Design review of the part built by this model. Coordinates are the model's own, in mm. A direction names the side the tool comes from. Round coordinates to 2 decimals unless told otherwise and drop trailing zeros. Order: outer loops, then holes, each group sorted by start corner. A loop starts at its lowest first (then second) coordinate and runs counter-clockwise, first axis right, second up. Notation, with made-up numbers: M 6,-20 L 41,-20 A29 ccw 41,12 Z; hole C -1.75,80 d5. An arc over 180 degrees is marked long. Write item = value, one per line. Start each with the question number.
```python
from build123d import *

# Parameters (mm, degrees)
F0_R     = 1.5875
F0_R_2   = 3.175
F1_DEPTH = 3.048


with BuildPart() as f1:
    # F0 (on Front) → F1 (new body)
    with BuildSketch(Plane.XZ):
        with BuildLine():
            ThreePointArc((45.0512324214, 0), (42.8445348199, 5.4919768863), (37.4514062495, 7.9303141575))
            ThreePointArc((37.4514062495, 7.9303141575), (29.1762324214, 0), (37.4514062495, -7.9303141575))
            ThreePointArc((37.4514062495, -7.9303141575), (42.8445348199, -5.4919768863), (45.0512324214, 0))
        make_face()
        with BuildLine():
            ThreePointArc((9.4553399063, 115.449857494), (9.507569027, 114.875982809), (9.525, 114.3))
            ThreePointArc((9.525, 114.3), (0.0975597085, 104.7754996402), (-9.5230014915, 114.1048908181))
            Line((-9.5230014915, 114.1048908181), (-15.7463614541, 65.5168604207))
            ThreePointArc((-15.7463614541, 65.5168604207), (0.016359288, 79.3749915708), (15.7504847833, 65.484402704))
            Line((15.7504847833, 65.484402704), (9.4553399063, 115.449857494))
        make_face()
        with Locations((-6.3508603799, 99.4688310552)):
            Circle(F0_R, mode=Mode.SUBTRACT)
        with BuildLine():
            ThreePointArc((15.875, 63.5), (15.8438406161, 64.4941526707), (15.7504847833, 65.484402704))
            ThreePointArc((15.7504847833, 65.484402704), (0.016359288, 79.3749915708), (-15.7463614541, 65.5168604207))
            ThreePointArc((-15.7463614541, 65.5168604207), (-15.8736111305, 63.7099873296), (-15.7942028036, 61.9003804205))
            ThreePointArc((-15.7942028036, 61.9003804205), (-0.1936293613, 47.6261809047), (15.7504847833, 61.515597296))
            ThreePointArc((15.7504847833, 61.515597296), (15.8438406161, 62.5058473293), (15.875, 63.5))
        make_face()
        with Locations((0, 63.5)):
            Circle(F0_R_2, mode=Mode.SUBTRACT)
        with BuildLine():
            ThreePointArc((-9.5230014915, 114.1048908181), (0.0975597085, 104.7754996402), (9.525, 114.3))
            ThreePointArc((9.525, 114.3), (9.507569027, 114.875982809), (9.4553399063, 115.449857494))
            ThreePointArc((9.4553399063, 115.449857494), (-0.6733337674, 123.8011708035), (-9.5230014915, 114.1048908181))
        make_face()
        with Locations((0, 114.3)):
            Circle(F0_R_2, mode=Mode.SUBTRACT)
        with BuildLine():
            ThreePointArc((15.7504847833, 61.515597296), (-0.1936293613, 47.6261809047), (-15.7942028036, 61.9003804205))
            Line((-15.7942028036, 61.9003804205), (-9.525, 0))
            ThreePointArc((-9.525, 0), (-6.7351920908, 6.7351920908), (0, 9.525))
            ThreePointArc((0, 9.525), (0.4052085937, 9.5163769889), (0.8096835142, 9.4905235686))
            ThreePointArc((0.8096835142, 9.4905235686), (7.0156204456, 6.4425689568), (9.525, 0))
            ThreePointArc((9.525, 0), (7.0156204456, -6.4425689568), (0.8096835142, -9.4905235686))
            Line((0.8096835142, -9.4905235686), (37.4514062495, -7.9303141575))
            ThreePointArc((37.4514062495, -7.9303141575), (29.1762324214, 0), (37.4514062495, 7.9303141575))
            Line((37.4514062495, 7.9303141575), (18.8646837389, 8.7217392657))
            ThreePointArc((18.8646837389, 8.7217392657), (13.1929762999, 11.4602704772), (11.2930893163, 17.4651225086))
            Line((11.2930893163, 17.4651225086), (15.7504847833, 61.515597296))
        make_face()
        with Locations((0, 63.5)):
            Circle(F0_R_2)
        with Locations((-6.3508603799, 99.4688310552)):
            Circle(F0_R)
        with BuildLine():
            ThreePointArc((0, 9.525), (-6.7351920908, 6.7351920908), (-9.525, 0))
            ThreePointArc((-9.525, 0), (-6.7351920908, -6.7351920908), (0, -9.525))
            Line((0, -9.525), (0.8096835142, -9.4905235686))
            ThreePointArc((0.8096835142, -9.4905235686), (7.0156204456, -6.4425689568), (9.525, 0))
            ThreePointArc((9.525, 0), (7.0156204456, 6.4425689568), (0.8096835142, 9.4905235686))
            Line((0.8096835142, 9.4905235686), (0, 9.525))
        make_face()
        with BuildLine():
            Line((0.8096835142, -9.4905235686), (0, -9.525))
            ThreePointArc((0, -9.525), (0.4052085937, -9.5163769889), (0.8096835142, -9.4905235686))
        make_face()
        with BuildLine():
            ThreePointArc((0.8096835142, 9.4905235686), (0.4052085937, 9.5163769889), (0, 9.525))
            Line((0, 9.525), (0.8096835142, 9.4905235686))
        make_face()
        with Locations((0, 114.3)):
            Circle(F0_R_2)
    extrude(amount=F1_DEPTH)


solid = f1.part
```
(1) For line 1 along Z through (x, y) = (-0.5, -0.5); line 2 along Z through (x, y) = (37, -2.5); line 3 along X through (y, z) = (-1.1, 64), list the stretches that pass through material, from the lowest coordinate up. Write a range as [from, to].
(2) Draft analysis for pull direction Z (two halves, no side actions). For faces 1 (the face through (28.29, -1.5, 8.32)), 2 (the face through (18.87, -1.5, -8.72)), 3 (the face through (13.253, -1.503, 11.392)), state which applies: pulls with the +Z half, pulls with the -Z half, needs draft (parallel to the pull), parting line crosses it, or undercut.
(3) Consider section C-C, the plane z = 33.5. Write out the cut boundary in (x, y).
(4) For faces 4 (the face through (13.49, -1.5, 39.18)), 5 (the face through (-12.703, -1.503, 31.383)), list the 3-axis set-ups (+Z, -Z, +X, -X, +Y, -Y) from which the entire face can be reached by the end or side of a thin tool; tool diameter is ignored.
(5) Consider section B-B, the plane x = 34.5. Write out the cut boundary in (y, z).
(6) Insertion check: pin 1 (1.5 mm diameter, centred on y = -2.5, z = 89.5, fed in from -X); pin 2 (1 mm diameter, centred on x = -6.5, y = -1.5, fed in from -Z). Each pin has a flat end and moves straight along its axis. Give the tip position at first contact, or say it passes through.
Completed:
q1.line_1 = [-9.51, 123.81]
q1.line_2 = [-7.95, 7.95]
q1.line_3 = [-15.87, 15.87]
q2.face_1 = pulls with the +Z half
q2.face_2 = pulls with the -Z half
q2.face_3 = undercut
q3.outline = M -12.92,-3.05 L 12.92,-3.05 L 12.92,0 L -12.92,0 Z
q4.face_4 = +X, +Y, -Y
q4.face_5 = -Z, -X, +Y, -Y
q5.outline = M -3.05,-8.06 L 0,-8.06 L 0,8.06 L -3.05,8.06 Z
q6.pin_1 = -12.77
q6.pin_2 = -7.4
